```python
from build123d import *

# Parameters (mm, degrees)
F0_R     = 1.25
F1_DEPTH = 3.5
F2_R     = 5
F3_R     = 2


with BuildPart() as f1:
    # F0 (on Front) → F1 (new body)
    with BuildSketch(Plane.XZ):
        with BuildLine():
            Line((15.646196, -1.805281), (15.75, 0))
            ThreePointArc((15.75, 0), (0, 15.75), (-15.75, 0))
            Line((-15.75, 0), (-15.646196, -1.805281))
            ThreePointArc((-15.646196, -1.805281), (0, -15.75), (15.646196, -1.805281))
        make_face()
        with BuildLine():
            ThreePointArc((-5.768629, -8.031371), (-8.031371, -8.031371), (-8.031371, -5.768629))
            Line((-8.031371, -5.768629), (-6.982024, -4.719283))
            ThreePointArc((-6.982024, -4.719283), (-4.719283, -4.719283), (-4.719283, -6.982024))
            Line((-4.719283, -6.982024), (-5.768629, -8.031371))
        make_face(mode=Mode.SUBTRACT)
        with BuildLine():
            ThreePointArc((-8.031371, 5.768629), (-8.031371, 8.031371), (-5.768629, 8.031371))
            Line((-5.768629, 8.031371), (-4.719283, 6.982024))
            ThreePointArc((-4.719283, 6.982024), (-4.719283, 4.719283), (-6.982024, 4.719283))
            Line((-6.982024, 4.719283), (-8.031371, 5.768629))
        make_face(mode=Mode.SUBTRACT)
        with BuildLine():
            Line((3.859728, 1.05), (7.45, 1.05))
            ThreePointArc((7.45, 1.05), (8.5, 0), (7.45, -1.05))
            Line((7.45, -1.05), (3.859728, -1.05))
            ThreePointArc((3.859728, -1.05), (2.828427, -2.828427), (1.05, -3.859728))
            Line((1.05, -3.859728), (1.05, -7.45))
            ThreePointArc((1.05, -7.45), (0, -8.5), (-1.05, -7.45))
            Line((-1.05, -7.45), (-1.05, -3.859728))
            ThreePointArc((-1.05, -3.859728), (-2.828427, -2.828427), (-3.859728, -1.05))
            Line((-3.859728, -1.05), (-7.45, -1.05))
            ThreePointArc((-7.45, -1.05), (-8.5, 0), (-7.45, 1.05))
            Line((-7.45, 1.05), (-3.859728, 1.05))
            ThreePointArc((-3.859728, 1.05), (-2.828427, 2.828427), (-1.05, 3.859728))
            Line((-1.05, 3.859728), (-1.05, 7.45))
            ThreePointArc((-1.05, 7.45), (0, 8.5), (1.05, 7.45))
            Line((1.05, 7.45), (1.05, 3.859728))
            ThreePointArc((1.05, 3.859728), (2.828427, 2.828427), (3.859728, 1.05))
        make_face(mode=Mode.SUBTRACT)
        with BuildLine():
            ThreePointArc((8.031371, -5.768629), (8.031371, -8.031371), (5.768629, -8.031371))
            Line((5.768629, -8.031371), (4.719283, -6.982024))
            ThreePointArc((4.719283, -6.982024), (4.719283, -4.719283), (6.982024, -4.719283))
            Line((6.982024, -4.719283), (8.031371, -5.768629))
        make_face(mode=Mode.SUBTRACT)
        with BuildLine():
            ThreePointArc((6.982024, 4.719283), (4.719283, 4.719283), (4.719283, 6.982024))
            Line((4.719283, 6.982024), (5.768629, 8.031371))
            ThreePointArc((5.768629, 8.031371), (8.031371, 8.031371), (8.031371, 5.768629))
            Line((8.031371, 5.768629), (6.982024, 4.719283))
        make_face(mode=Mode.SUBTRACT)
        with BuildLine():
            ThreePointArc((15.646196, -1.805281), (15.724028, -0.904132), (15.75, 0))
            Line((15.75, 0), (15.646196, -1.805281))
        make_face()
        with BuildLine():
            Line((-15.646196, -1.805281), (-15.75, 0))
            ThreePointArc((-15.75, 0), (-15.724028, -0.904132), (-15.646196, -1.805281))
        make_face()
        with BuildLine():
            Line((10, -100), (15.646196, -1.805281))
            ThreePointArc((15.646196, -1.805281), (0, -15.75), (-15.646196, -1.805281))
            Line((-15.646196, -1.805281), (-10, -100))
            Line((-10, -100), (0, -100))
            Line((0, -100), (10, -100))
        make_face()
        with Locations((0, -95)):
            Circle(F0_R, mode=Mode.SUBTRACT)
        with Locations((0, -87)):
            Circle(F0_R, mode=Mode.SUBTRACT)
        Polygon((-8.892545, -67), (0, -67), (8.892545, -67), (8.173795, -79.5), (0, -79.5), (-8.173795, -79.5), align=None, mode=Mode.SUBTRACT)
        Polygon((-10.215045, -44), (0, -44), (10.215045, -44), (9.180045, -62), (0, -62), (-9.180045, -62), align=None, mode=Mode.SUBTRACT)
        Polygon((-11.69567, -18.25), (0, -18.25), (11.69567, -18.25), (10.502545, -39), (0, -39), (-10.502545, -39), align=None, mode=Mode.SUBTRACT)
    extrude(amount=F1_DEPTH)

    # F2
    f2_edges = [f1.edges().sort_by_distance(p)[0] for p in [
        (-10, -1.75, -100),
        (10, -1.75, -100),
    ]]
    fillet(f2_edges, radius=F2_R)

    # F3
    f3_edges = [f1.edges().sort_by_distance(p)[0] for p in [
        (-10.502545, -1.75, -39),
        (-9.180045, -1.75, -62),
        (-8.173795, -1.75, -79.5),
        (-8.892545, -1.75, -67),
        (-10.215045, -1.75, -44),
        (-11.69567, -1.75, -18.25),
        (11.69567, -1.75, -18.25),
        (10.215045, -1.75, -44),
        (8.892545, -1.75, -67),
        (10.502545, -1.75, -39),
        (9.180045, -1.75, -62),
        (8.173795, -1.75, -79.5),
    ]]
    fillet(f3_edges, radius=F3_R)


solid = f1.part
```
CAD build for the part. Positions are in the model's coordinates, mm. Give positions to 0.01 mm unless a question says otherwise; leave off trailing zeros. Order: outer loops, then holes, each group sorted by start corner. A loop starts at its lowest first (then second) coordinate and runs counter-clockwise, first axis right, second up. Notation, with made-up numbers: M -10,68.5 L 49,68.5 A4 cw 49,73.5 Z; hole C 20.5,66 d3. An arc over 180 degrees is marked long. Put each result on its own line as item: value. Start each with the question number.
(1) Mould opens along X. For faces 1 (the cylindrical face through (8.673, -1.774, -98.672)), 2 (the cylindrical face through (-0.16, -1.73, -85.76)), 3 (the cylindrical face through (-10, -1.77, -38.44)), 4 (the cylindrical face through (-15.725, -1.726, -0.891)) say: +X half, -X half, draft (parallel to the pull), parting line (faces both ways), or undercut.
(2) Saw through at C-C, the plane y = -2.2. Give the number of separate pieces and of enclosed holes in the cut face, then the cut area to 3 significant figures.
(3) Saw through at D-D, the plane z = -91.5. Write the cut outline in (x, y), then the cut area to 3 significant figures.
(4) Flat gauge pins, fed straight in: pin 1 Ø1 at (y, z) = (-1.5, -5.5) entering from -X; pin 2 Ø1.8 at (y, z) = (-2.5, 5.5) entering from +X; pin 3 Ø1 at (x, y) = (-1.5, -1) entering from +Z; pin 4 Ø1 at (x, z) = (-9.5, -40.5) entering from +Y. Where does each tip first touch, or does it go through?
(5) Saw through at B-B, the plane z = -55. Write the cut outline in (x, y), then the cut area to 3 significant figures.
(6) Saw through at A-A, the plane x = 0. Write the cut outline in (y, z).
(7) Drill centre lines: line 1 along X through (y, z) = (-1.9, -95); line 2 along Z through (x, y) = (-4, -1.6); line 3 along Z through (x, y) = (1.5, -2.15). Where is each one in solid material? Low to high.
Check result:
1. face 1: +X half
1. face 2: undercut
1. face 3: undercut
1. face 4: -X half
2. separate pieces: 1
2. enclosed holes: 10
2. area: 1,800 mm2
3. outline: M -10.49,-3.5 L 10.49,-3.5 L 10.49,0 L -10.49,0 Z
3. area: 73.4 mm2
4. pin 1: stops at x = -15.46
4. pin 2: stops at x = 15.06
4. pin 3: stops at z = 15.72
4. pin 4: stops at y = 0
5. outline: M -12.59,-3.5 L -9.58,-3.5 L -9.58,0 L -12.59,0 Z; M 9.58,-3.5 L 12.59,-3.5 L 12.59,0 L 9.58,0 Z
5. area: 21.0 mm2
6. outline: M -3.5,-100 L 0,-100 L 0,-96.25 L -3.5,-96.25 Z; M -3.5,-93.75 L 0,-93.75 L 0,-88.25 L -3.5,-88.25 Z; M -3.5,-85.75 L 0,-85.75 L 0,-79.5 L -3.5,-79.5 Z; M -3.5,-67 L 0,-67 L 0,-62 L -3.5,-62 Z; M -3.5,-44 L 0,-44 L 0,-39 L -3.5,-39 Z; M -3.5,-18.25 L 0,-18.25 L 0,-8.5 L -3.5,-8.5 Z; M -3.5,8.5 L 0,8.5 L 0,15.75 L -3.5,15.75 Z
7. line 1: x = -10.29 to -1.25, 1.25 to 10.29
7. line 2: z = -100 to -79.5, -67 to -62, -44 to -39, -18.25 to -1.05, 1.05 to 15.23
7. line 3: z = -100 to -79.5, -67 to -62, -44 to -39, -18.25 to -3.71, 3.71 to 15.68
